Study the drawing (mm; zero at the part's minimum x, y, z) and answer. A direction names the side the tool comes from. Give positions to 0.01 mm unless a question says otherwise; leave off trailing zeros. Order: outer loops, then holes, each group sorted by start corner. A loop starts at its lowest first (then second) coordinate and runs counter-clockwise, first axis right, second up.
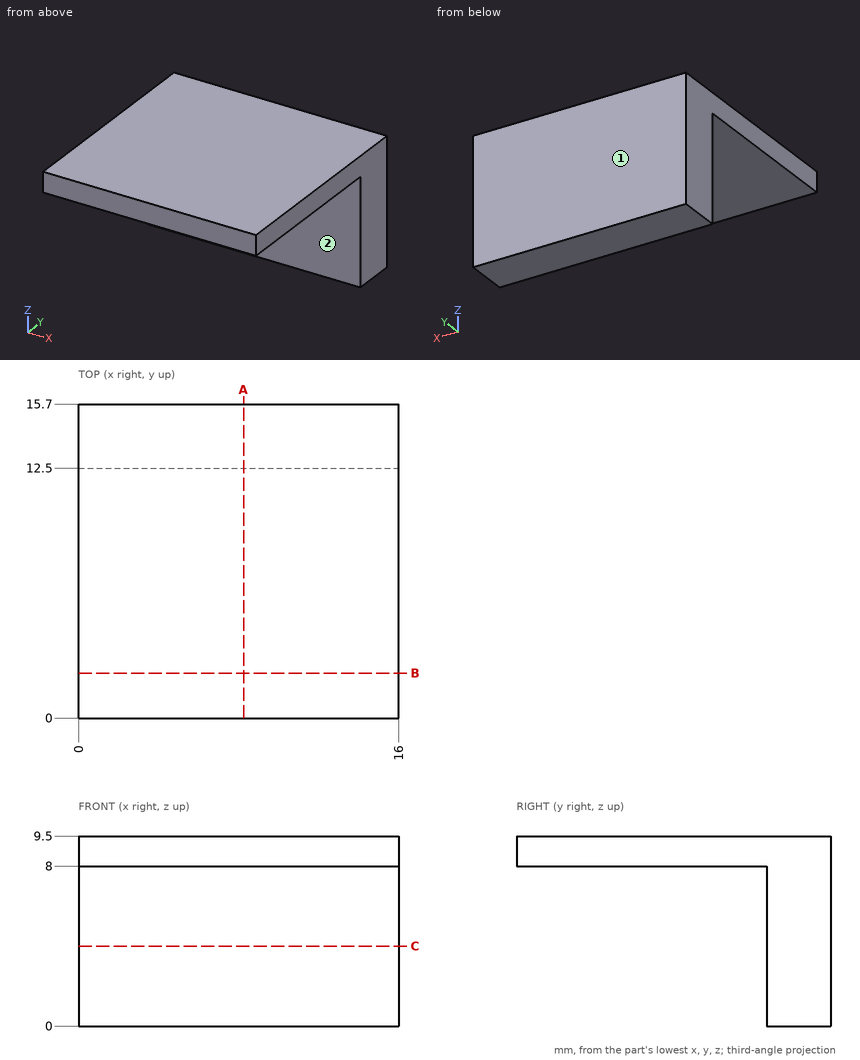
1) Find section C-C (z = 4). Write down the section's boundary in (x, y), then the cut area to 3 significant figures.
Geometry says:
outline: (0, 12.5) - (16, 12.5) - (16, 15.7) - (0, 15.7) - close
area: 51.2 mm2
2) A tool of negligible diameter and unlimited length cuts with its end or side. For the marked faces 1 and 2, from which of +Z, -Z, +X, -X, +Y, -Y can it reach the whole face along a straight path? Write none if from no direction.
Geometry says:
face 1: +Z, -Z, +X, -X, +Y
face 2: -Z, +X, -X, -Y
3) Find section B-B (y = 2.25). Write down the section's boundary in (x, z), then the cut area to 3 significant figures.
Geometry says:
outline: (0, 8) - (16, 8) - (16, 9.5) - (0, 9.5) - close
area: 24.0 mm2
4) Find section A-A (x = 8.25). Write down the section's boundary in (y, z).
Geometry says:
outline: (0, 8) - (12.5, 8) - (12.5, 0) - (15.7, 0) - (15.7, 9.5) - (0, 9.5) - close
5) Straight lines are drawn through the part: probe 1 along Z at (x, y) = (12.5, 10.5); probe 2 along Y at (x, z) = (4, 3). For each, find the intervals that lie inside material, in ascending order.
Geometry says:
probe 1: z = 8 to 9.5
probe 2: y = 12.5 to 15.7
6) Given P1, Ø3, axis at x = 12.5, y = 9.5, coming from the -Z side; P2, Ø4, axis at x = 11, z = 4, coming from the -Y side, each flat-ended and moving along its own axis, determine where each tip first touches the part or whether it passes through.
Geometry says:
P1: stops at z = 8
P2: stops at y = 12.5
